from build123d import *

# Parameters (mm, degrees)
SKETCH_1_W          = 9
SKETCH_1_H          = 9
SKETCH_1_W_2        = 7
SKETCH_1_H_2        = 7
EXTRUDE_1_DEPTH     = 70
CUT_EXTRUDE_1_DEPTH = 100
SKETCH_3_R          = 1.6
CUT_EXTRUDE_2_DEPTH = 100
SKETCH_4_R          = 1.6
CUT_EXTRUDE_3_DEPTH = 100
SKETCH_5_R          = 1.6
CUT_EXTRUDE_4_DEPTH = 10
SKETCH_6_W          = 9
SKETCH_6_H          = 9
SKETCH_6_W_2        = 7
SKETCH_6_H_2        = 7
EXTRUDE_2_DEPTH     = 5


with BuildPart() as part:
    # ｽｹｯﾁ1 → ﾎﾞｽ - 押し出し1 (new body)
    with BuildSketch(Plane.XY):
        Rectangle(SKETCH_1_W, SKETCH_1_H)
        Rectangle(SKETCH_1_W_2, SKETCH_1_H_2, mode=Mode.SUBTRACT)
    extrude(amount=EXTRUDE_1_DEPTH)

    # ｽｹｯﾁ2 → ｶｯﾄ - 押し出し1 (cut)
    with BuildSketch(Plane(origin=(0, 4.5, 0), x_dir=(1, 0, 0), z_dir=(0, 1, 0))):
        with BuildLine():
            ThreePointArc((2.5, -10), (1.767766953, -8.232233047), (0, -7.5))
            Line((0, -7.5), (0, -10))
            Line((0, -10), (0, -12.5))
            ThreePointArc((0, -12.5), (1.767766953, -11.767766953), (2.5, -10))
        make_face()
        with BuildLine():
            Line((0, -10), (0, -7.5))
            ThreePointArc((0, -7.5), (-2.5, -10), (0, -12.5))
            Line((0, -12.5), (0, -10))
        make_face()
    extrude(amount=-CUT_EXTRUDE_1_DEPTH, mode=Mode.SUBTRACT)

    # ｽｹｯﾁ3 → ｶｯﾄ - 押し出し2 (cut)
    with BuildSketch(Plane(origin=(0, 4.5, 0), x_dir=(1, 0, 0), z_dir=(0, 1, 0))):
        with Locations((0, -3)):
            Circle(SKETCH_3_R)
    extrude(amount=-CUT_EXTRUDE_2_DEPTH, mode=Mode.SUBTRACT)

    # ｽｹｯﾁ4 → ｶｯﾄ - 押し出し3 (cut)
    with BuildSketch(Plane(origin=(0, 4.5, 0), x_dir=(1, 0, 0), z_dir=(0, 1, 0))):
        with Locations((0, -65.5)):
            Circle(SKETCH_4_R)
        with Locations((0, -55.5)):
            Circle(SKETCH_4_R)
    extrude(amount=-CUT_EXTRUDE_3_DEPTH, mode=Mode.SUBTRACT)

    # ｽｹｯﾁ5 → ｶｯﾄ - 押し出し4 (cut, through all)
    with BuildSketch(Plane(origin=(0, 4.5, 0), x_dir=(1, 0, 0), z_dir=(0, 1, 0))):
        with Locations((0, -35)):
            Circle(SKETCH_5_R)
    extrude(amount=-CUT_EXTRUDE_4_DEPTH, mode=Mode.SUBTRACT)

    # ｽｹｯﾁ6 → ﾎﾞｽ - 押し出し2 (add)
    with BuildSketch(Plane(origin=(0, 0, 0), x_dir=(-1, 0, 0), z_dir=(0, 0, -1))):
        Rectangle(SKETCH_6_W, SKETCH_6_H)
        Rectangle(SKETCH_6_W_2, SKETCH_6_H_2, mode=Mode.SUBTRACT)
    extrude(amount=EXTRUDE_2_DEPTH)


solid = part.part
Read the model definition and answer for the solid it produces. Units are mm, in the model's axes. A direction names the side the tool comes from. Round coordinates to 2 decimals unless told otherwise and drop trailing zeros. Order: outer loops, then holes, each group sorted by start corner. A loop starts at its lowest first (then second) coordinate and runs counter-clockwise, first axis right, second up. Notation, with made-up numbers: (-12.75, -21) - (36.25, -21) arc R14 ccw to (36.25, 0) - close; hole circle Ø1 at (-14, 80). An arc over 180 degrees is marked (long way). Use one line per item in the form item = value. Start each with the question number.
(1) Determine the mould class of faces 3 (the face through (-4.5, 0, 33)), 4 (the face through (-0.208, 4.007, 63.914)), 5 (the face through (0, -4.5, 33)) for opening direction X: +X half, -X half, draft (parallel to the pull), parting line (faces both ways), or undercut.
(2) For faces 1 (the face through (0, -3.5, 33)), 2 (the face through (-0.35, -3.99, 4.56)), determine the directions among +Z, -Z, +X, -X, +Y, -Y from which every point of the face is accessible in a straight line to the end or side of a thin tool.
(3) The part is cut by section C-C (z = 35). Give the vertices of the cut face in (x, y), then the cut area to 3 significant figures.
(4) The part is cut by section B-B (y = 1.25). Give the vertices of the cut face in (x, z), then the cut area to 3 significant figures.
(5) The part is cut by section A-A (z = 5.5). Give the vertices of the cut face in (x, y).
(6) Find the intervals of material crossed by line 1 along Z through (x, y) = (0, -3.7); line 2 along X through (y, z) = (-0.25, 55); line 3 along X through (y, z) = (-3.8, 35), in increasing order. Write a range as from..to.
Checked values:
q1.face_3 = -X half
q1.face_4 = undercut
q1.face_5 = draft
q2.face_1 = +Z, -Z
q2.face_2 = +Y, -Y
q3.outline = (-4.5, -4.5) - (-1.6, -4.5) - (-1.6, -3.5) - (-3.5, -3.5) - (-3.5, 3.5) - (-1.6, 3.5) - (-1.6, 4.5) - (-4.5, 4.5) - close; (1.6, -4.5) - (4.5, -4.5) - (4.5, 4.5) - (1.6, 4.5) - (1.6, 3.5) - (3.5, 3.5) - (3.5, -3.5) - (1.6, -3.5) - close
q3.area = 25.6 mm^2
q4.outline = (-4.5, -5) - (-3.5, -5) - (-3.5, 70) - (-4.5, 70) - close; (3.5, -5) - (4.5, -5) - (4.5, 70) - (3.5, 70) - close
q4.area = 150 mm^2
q5.outline = (-4.5, -4.5) - (4.5, -4.5) - (4.5, 4.5) - (-4.5, 4.5) - close; hole (-3.5, -3.5) - (3.5, -3.5) - (3.5, 3.5) - (-3.5, 3.5) - close
q6.line_1 = -5..1.4, 4.6..7.5, 12.5..33.4, 36.6..53.9, 57.1..63.9, 67.1..70
q6.line_2 = -4.5..-3.5, 3.5..4.5
q6.line_3 = -4.5..-1.6, 1.6..4.5
